```python
from build123d import *

# Parameters (mm, degrees)
BOSS_EXTRUDE1_DEPTH = 228.6
SKETCH3_R           = 2.413
CUT_EXTRUDE1_DEPTH  = 1.905
LPATTERN1_COUNT     = 3
LPATTERN1_PITCH     = 76.2
CUT_EXTRUDE3_DEPTH  = 230.107436806
FILLET1_R           = 2.54


with BuildPart() as part:
    # Sketch2 → Boss-Extrude1 (new, symmetric)
    with BuildSketch(Plane(origin=(0, 0, 0), x_dir=(0, 0, -1), z_dir=(1, 0, 0))):
        Polygon((0, 9.144), (-12.192, 9.144), (-12.192, 4.445), (-10.6045, 4.445), (-10.6045, 5.969), (-4.2545, 5.969), (-4.2545, 4.445), (-1.905, 4.445), (-1.905, -4.445), (-4.2545, -4.445), (-4.2545, -5.969), (-10.6045, -5.969), (-10.6045, -4.445), (-12.192, -4.445), (-12.192, -9.144), (0, -9.144), align=None)
    extrude(amount=BOSS_EXTRUDE1_DEPTH, both=True)

    # Sketch3 → Cut-Extrude1 (cut)
    with BuildSketch(Plane.XY.offset(1.905)):
        with Locations((38.1, 0)):
            Circle(SKETCH3_R)
    cut_extrude1 = extrude(amount=-CUT_EXTRUDE1_DEPTH, mode=Mode.SUBTRACT)

    # LPattern1: Cut-Extrude1 ×3
    with Locations(*[(i * LPATTERN1_PITCH, 0, 0) for i in range(1, LPATTERN1_COUNT)]):
        add(cut_extrude1, mode=Mode.SUBTRACT)

    # SurfaceCut1
    split(bisect_by=Plane(origin=(0, 0, 0), x_dir=(0, 0, -1), z_dir=(1, 0, 0)), keep=Keep.TOP)

    # Mirror1: part across plane


with BuildPart() as part_1:
    add(part.part)
    add(part.part.mirror(Plane(origin=(0, 0, 0), x_dir=(0, 0, 1), z_dir=(1, 0, 0))))

    # Sketch4 → Cut-Extrude3 (cut, through all)
    with BuildSketch(Plane.XY.offset(12.192)):
        Polygon((-209.55, -9.144), (-191.262, 9.144), (-228.6, 9.144), (-228.6, -9.144), align=None)
    extrude(amount=-CUT_EXTRUDE3_DEPTH, mode=Mode.SUBTRACT)

    # Fillet1
    # the kernel refuses this fillet: 2.54 mm, written as the material it takes off along each edge
    with BuildSketch(Plane(origin=(-209.55, -9.144, 27.522256121), x_dir=(0.7071067811865455, 0.7071067811865496, 0), z_dir=(0, 0, -1))) as fillet1_piece_1:
        with BuildLine():
            CenterArc((FILLET1_R * 2.41421356237, FILLET1_R), FILLET1_R, 135, 135)
            Line((FILLET1_R * 1.70710678119, FILLET1_R * 1.70710678119), (0, 0))
            Line((0, 0), (FILLET1_R * 2.41421356237, 0))
        make_face()
    extrude(amount=42.852512242, mode=Mode.SUBTRACT)


solid = part_1.part
```
The model under review builds one solid part; all positions refer to its coordinate system, in mm. Round coordinates to 2 decimals unless told otherwise and drop trailing zeros. Loops run counter-clockwise (first coordinate to the right, second up) from the corner with the lowest first, then second, coordinate; pieces in that order, holes last.
Item 1: Clearance check with a flat-ended pin moving along its axis: pin 1 Ø5.5 at (x, y) = (38.1, 0) entering from +Z (3 decimals). State where the tip first meets the part, or that it passes through.
Determined:
pin 1: stops at z = 1.905
Item 2: For line 1 (Y direction, x = -114.3, z = 1.35); line 2 (Y direction, x = 163.5, z = 9.5); line 3 (Z direction, x = 48, y = -1.75) (3 decimals), list the stretches that pass through material, from the lowest coordinate up.
Determined:
line 1: y = -9.14 to -2.41, 2.41 to 9.14
line 2: y = -9.14 to -5.97, 5.97 to 9.14
line 3: z = 0 to 1.905
Item 3: Take a section at A-A (x = 67). Write out the cut boundary in (y, z) (1 decimal), then the cut area to 3 significant figures.
Determined:
outline: (-9.1, 0) - (9.1, 0) - (9.1, 12.2) - (4.4, 12.2) - (4.4, 10.6) - (6, 10.6) - (6, 4.3) - (4.4, 4.3) - (4.4, 1.9) - (-4.4, 1.9) - (-4.4, 4.3) - (-6, 4.3) - (-6, 10.6) - (-4.4, 10.6) - (-4.4, 12.2) - (-9.1, 12.2) - close
area: 112 mm2
Item 4: Mouldability with a two-part tool opening along Y and no side actions: class faces 1 (the face through (8, 0, 0)), 2 (the face through (9, 0, 1.905)), 3 (the face through (16, 9.144, 6)) as released by +Y, released by -Y, zero draft, split by the parting line, or undercut.
Determined:
face 1: zero draft
face 2: undercut
face 3: released by +Y
